Part model, mm, in its own coordinate system. Round coordinates to 2 decimals unless told otherwise and drop trailing zeros. Loops run counter-clockwise (first coordinate to the right, second up) from the corner with the lowest first, then second, coordinate; pieces in that order, holes last.
1) Band-saw the part on A-A, the plane z = 0. Write the cut outline in (x, y) (1 decimal).
2) Band-saw the part on C-C, the plane y = 0.85. State how many separate pieces and enclosed holes the cut face has, then the cut area to 3 significant figures.
3) Probe line 1 (X direction, y = 1.1, z = 0) (1 decimal); line 2 (Z direction, x = -45.5, y = 0.35); line 3 (Z direction, x = -39.5, y = 1.45). List the from-to ranges inside material, lowest first.
4) Drop flat-ended pins along their axis: P1, Ø3, axis at x = 8.33, z = 0, coming from the +Y side; P2, Ø0.8, axis at y = 1, z = 34, coming from the +X side. Give the stop position or say it passes through.
5) Band-saw the part on B-B, the plane z = 29. Write the cut outline in (x, y).
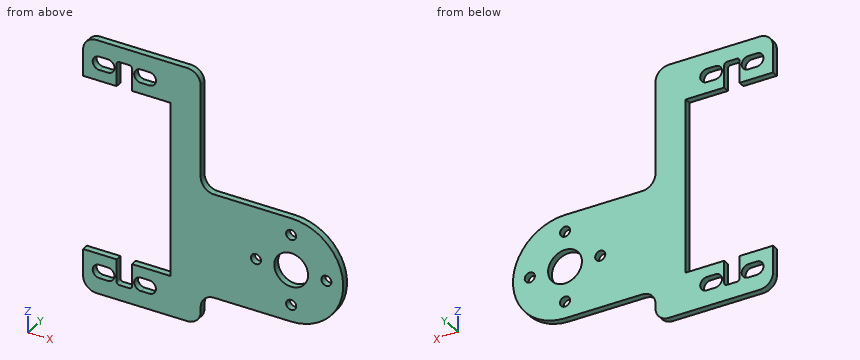
from build123d import *

# Parameters (mm, degrees)
SKETCH1_R          = 4.0005
SKETCH1_R_2        = 1.1938
BASE_FLANGE1_DEPTH = 1.524
SKETCH3_W          = 20.6756
SKETCH3_H          = 41.275
EXTRUDE1_DEPTH     = 1.524
SKETCH4_W          = 3.6195
SKETCH4_H          = 5.9436
EXTRUDE2_DEPTH     = 1.524
FILLET1_R          = 3.175
FILLET2_RADIUS     = 12.3063
FILLET2_LENGTH     = 1.524
FILLET3_R          = 0.635


# Sheet-metal steps are written as plain solids
with BuildPart() as part:
    # Sketch1 → Base-Flange1 (new body)
    with BuildSketch(Plane(origin=(0, 0, 0), x_dir=(1, 0, 0), z_dir=(0, 1, 0))):
        Polygon((12.3063, 12.3063), (12.3063, -12.3063), (-21.3995, -12.3063), (-21.3995, -40.4749), (-49.2125, -40.4749), (-49.2125, 19.8501), (-21.3995, 19.8501), (-21.3995, 12.3063), align=None)
        with Locations(Location((0, 0, 0), (0, 0, 90))):
            Circle(SKETCH1_R, mode=Mode.SUBTRACT)
        with Locations(Location((0, 8.3312, 0), (0, 0, 90))):
            Circle(SKETCH1_R_2, mode=Mode.SUBTRACT)
        with Locations(Location((8.3312, 0, 0), (0, 0, 90))):
            Circle(SKETCH1_R_2, mode=Mode.SUBTRACT)
        with Locations(Location((0, -8.3312, 0), (0, 0, 90))):
            Circle(SKETCH1_R_2, mode=Mode.SUBTRACT)
        with Locations(Location((-8.3312, 0, 0), (0, 0, 90))):
            Circle(SKETCH1_R_2, mode=Mode.SUBTRACT)
    extrude(amount=BASE_FLANGE1_DEPTH)

    # Sketch3 → Extrude1 (cut)
    with BuildSketch(Plane(origin=(0, 1.524, 0), x_dir=(1, 0, 0), z_dir=(0, 1, 0))):
        with Locations((-38.8747, -10.3124)):
            Rectangle(SKETCH3_W, SKETCH3_H)
    extrude(amount=-EXTRUDE1_DEPTH, mode=Mode.SUBTRACT)

    # Sketch4 → Extrude2 (cut)
    with BuildSketch(Plane(origin=(0, 1.524, 0), x_dir=(1, 0, 0), z_dir=(0, 1, 0))):
        with Locations((-39.46525, 13.2969)):
            Rectangle(SKETCH4_W, SKETCH4_H)
        with Locations((-39.46525, -33.9217)):
            Rectangle(SKETCH4_W, SKETCH4_H)
        with BuildLine():
            Line((-35.5473, 16.0782), (-33.5661, 16.0782))
            ThreePointArc((-33.5661, 16.0782), (-31.9786, 14.4907), (-33.5661, 12.9032))
            Line((-33.5661, 12.9032), (-35.5473, 12.9032))
            ThreePointArc((-35.5473, 12.9032), (-37.1348, 14.4907), (-35.5473, 16.0782))
        make_face()
        with BuildLine():
            Line((-45.3517, 16.0782), (-43.3705, 16.0782))
            ThreePointArc((-43.3705, 16.0782), (-41.783, 14.4907), (-43.3705, 12.9032))
            Line((-43.3705, 12.9032), (-45.3517, 12.9032))
            ThreePointArc((-45.3517, 12.9032), (-46.9392, 14.4907), (-45.3517, 16.0782))
        make_face()
        with BuildLine():
            Line((-35.5473, -33.528), (-33.5661, -33.528))
            ThreePointArc((-33.5661, -33.528), (-31.9786, -35.1155), (-33.5661, -36.703))
            Line((-33.5661, -36.703), (-35.5473, -36.703))
            ThreePointArc((-35.5473, -36.703), (-37.1348, -35.1155), (-35.5473, -33.528))
        make_face()
        with BuildLine():
            Line((-45.3517, -33.528), (-43.3705, -33.528))
            ThreePointArc((-43.3705, -33.528), (-41.783, -35.1155), (-43.3705, -36.703))
            Line((-43.3705, -36.703), (-45.3517, -36.703))
            ThreePointArc((-45.3517, -36.703), (-46.9392, -35.1155), (-45.3517, -33.528))
        make_face()
    extrude(amount=-EXTRUDE2_DEPTH, mode=Mode.SUBTRACT)

    # Fillet1
    fillet1_edges = [part.edges().sort_by_distance(p)[0] for p in [
        (-21.3995, 0.762, 12.3063),
        (-21.3995, 0.762, 40.4749),
        (-49.2125, 0.762, 40.4749),
        (-49.2125, 0.762, -19.8501),
        (-21.3995, 0.762, -19.8501),
        (-21.3995, 0.762, -12.3063),
    ]]
    fillet(fillet1_edges, radius=FILLET1_R)

    # Fillet2: full round fillet: the end face becomes a half cylinder, R = half its width
    fillet2_face = Plane((12.3063, 0.762, 0), x_dir=(0, 1, 0), z_dir=(1, 0, 0))  # on the end face: x along it, z out of the body
    fillet2_slab = fillet2_face.offset(-FILLET2_RADIUS / 2) * Box(FILLET2_LENGTH, 2 * FILLET2_RADIUS, FILLET2_RADIUS, mode=Mode.PRIVATE)  # the body's end, R deep
    fillet2_round = Plane((0, 0.762, 0), x_dir=(1, 0, 0), z_dir=(0, 1, 0)) * Cylinder(FILLET2_RADIUS, FILLET2_LENGTH, mode=Mode.PRIVATE)  # its axis R under the face
    add(fillet2_slab - fillet2_round, mode=Mode.SUBTRACT)

    # Fillet3
    fillet3_edges = [part.edges().sort_by_distance(p)[0] for p in [
        (-41.275, 0.762, -16.2687),
        (-37.6555, 0.762, -16.2687),
        (-41.275, 0.762, 36.8935),
        (-37.6555, 0.762, 36.8935),
    ]]
    fillet(fillet3_edges, radius=FILLET3_R)


solid = part.part
Reported:
1. outline: (-28.5, 0) - (-9.5, 0) - (-9.5, 1.5) - (-28.5, 1.5) - close; (-7.1, 0) - (-4, 0) - (-4, 1.5) - (-7.1, 1.5) - close; (4, 0) - (7.1, 0) - (7.1, 1.5) - (4, 1.5) - close; (9.5, 0) - (12.3, 0) - (12.3, 1.5) - (9.5, 1.5) - close
2. separate pieces: 1
2. enclosed holes: 9
2. area: 1,420 mm2
3. line 1: x = -28.5 to -9.5, -7.1 to -4, 4 to 7.1, 9.5 to 12.3
3. line 2: z = -19.85 to -16.07, -12.91 to -10.33, 30.95 to 33.53, 36.7 to 40.47
3. line 3: z = -19.85 to -16.27, 36.89 to 40.47
4. P1: stops at y = 1.52
4. P2: stops at x = -21.4
5. outline: (-28.54, 0) - (-21.4, 0) - (-21.4, 1.52) - (-28.54, 1.52) - close
